Could you check a few things on this drawing? It's one solid part, dimensions in mm from its lowest x, y, z. A direction names the side the tool comes from. Give positions to 0.01 mm unless a question says otherwise; leave off trailing zeros. Loops run counter-clockwise (first coordinate to the right, second up) from the corner with the lowest first, then second, coordinate; pieces in that order, holes last.
1. For P1, Ø2, axis at y = 3, z = 22, coming from the +X side; P2, Ø10, axis at y = 7.5, z = 27.5, coming from the -X side; P3, Ø1.5, axis at x = 6.5, y = 10, coming from the +Z side, each with a flat end and sliding along its axis, tell me the tip position at first contact or that it passes through.
2. I need wall thicknesses on line 1 along Z through (x, y) = (13, 13); line 2 along Y through (x, z) = (16.75, 30); line 3 along Z through (x, y) = (8.5, 19.75). Which ranges of each line are inside material? Lowest first, please.
3. Imagine slicing it at A-A (y = 13). List the corners of the cut face in (x, z) for me, plus the area to 3 significant figures.
4. Imagine slicing it at D-D (x = 27). List the corners of the cut face in (y, z) for me, plus the area to 3 significant figures.
5. Imagine slicing it at B-B (z = 30). List the corners of the cut face in (x, y) for me, plus the area to 3 significant figures.
6. For the marked faces 4, 5 and 6, which set-ups out of +Z, -Z, +X, -X, +Y, -Y let a thin tool reach every point of the face, with its end or its side?
7. Imagine slicing it at C-C (y = 18.5). List the corners of the cut face in (x, z) for me.
8. Thinking about a two-plate mould opening in Z: for the marked faces 1, 2 and 3, which applies, +Z half, -Z half, draft (parallel to the pull), parting line (faces both ways), or undercut?
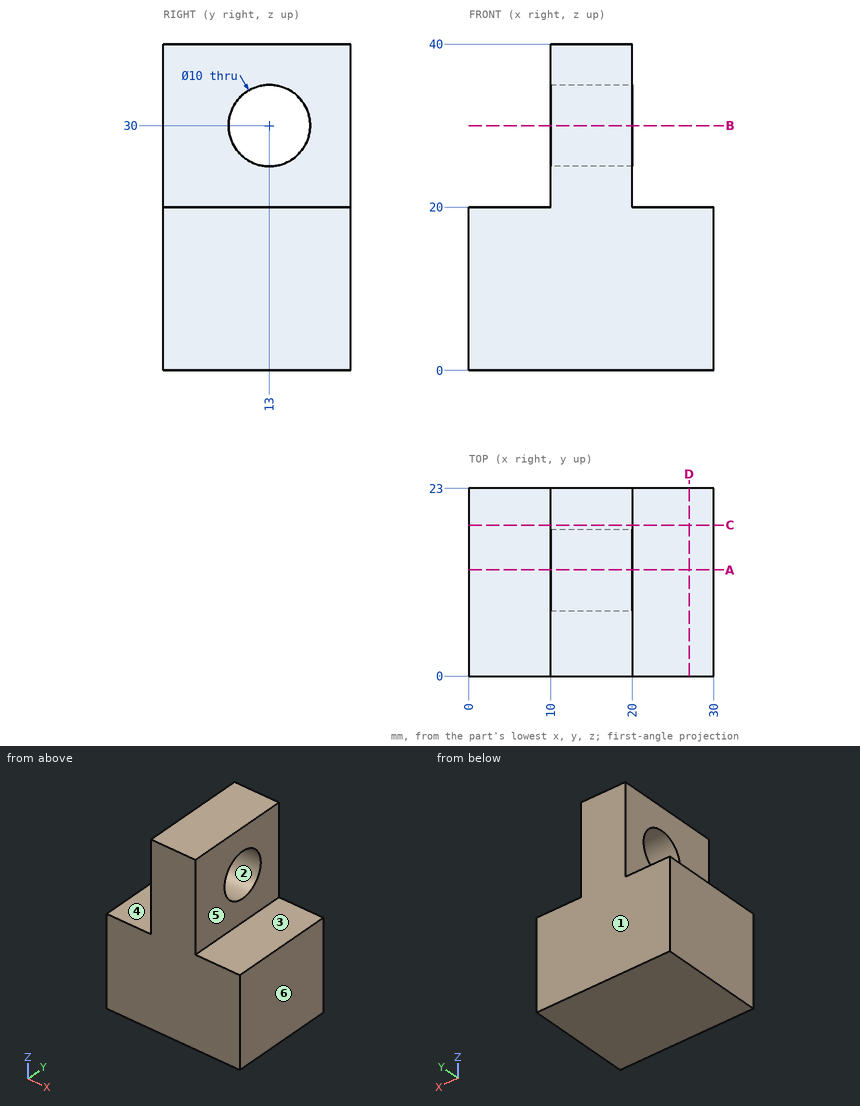
Derived:
1. P1: stops at x = 20
1. P2: stops at x = 10
1. P3: stops at z = 20
2. line 1: z = 0 to 25, 35 to 40
2. line 2: y = 0 to 8, 18 to 23
2. line 3: z = 0 to 20
3. outline: (0, 0) - (30, 0) - (30, 20) - (20, 20) - (20, 25) - (10, 25) - (10, 20) - (0, 20) - close; (10, 35) - (20, 35) - (20, 40) - (10, 40) - close
3. area: 700 mm2
4. outline: (0, 0) - (23, 0) - (23, 20) - (0, 20) - close
4. area: 460 mm2
5. outline: (10, 0) - (20, 0) - (20, 8) - (10, 8) - close; (10, 18) - (20, 18) - (20, 23) - (10, 23) - close
5. area: 130 mm2
6. face 4: +Z, -X, +Y, -Y
6. face 5: +Z, +X, +Y, -Y
6. face 6: +Z, -Z, +X, +Y, -Y
7. outline: (0, 0) - (30, 0) - (30, 20) - (20, 20) - (20, 40) - (10, 40) - (10, 20) - (0, 20) - close
8. face 1: draft
8. face 2: undercut
8. face 3: +Z half
